from build123d import *

# Parameters (mm, degrees)
MODEL_R                 = 1.5
SALIENTE_EXTRUIR1_DEPTH = 3


with BuildPart() as part:
    # Model → Saliente-Extruir1 (new body)
    with BuildSketch(Plane.XY):
        with BuildLine():
            Line((-105.943383637, 101.056539338), (-105.943383637, 65.056539338))
            ThreePointArc((-105.943383637, 65.056539338), (-104.625364152, 61.874558823), (-101.443383637, 60.556539338))
            Line((-101.443383637, 60.556539338), (-83.443383637, 60.556539338))
            ThreePointArc((-83.443383637, 60.556539338), (-80.261403122, 61.874558823), (-78.943383637, 65.056539338))
            Line((-78.943383637, 65.056539338), (-78.943383637, 101.056539338))
            ThreePointArc((-78.943383637, 101.056539338), (-80.261403122, 104.238519853), (-83.443383637, 105.556539338))
            Line((-83.443383637, 105.556539338), (-101.443383637, 105.556539338))
            ThreePointArc((-101.443383637, 105.556539338), (-104.625364152, 104.238519853), (-105.943383637, 101.056539338))
        make_face()
        with Locations((-101.443383637, 101.056539338)):
            Circle(MODEL_R, mode=Mode.SUBTRACT)
        with Locations((-92.443383637, 101.056539338)):
            Circle(MODEL_R, mode=Mode.SUBTRACT)
        with Locations((-83.443383637, 101.056539338)):
            Circle(MODEL_R, mode=Mode.SUBTRACT)
        with Locations((-101.443383637, 92.056539338)):
            Circle(MODEL_R, mode=Mode.SUBTRACT)
        with Locations((-92.443383637, 92.056539338)):
            Circle(MODEL_R, mode=Mode.SUBTRACT)
        with Locations((-83.443383637, 92.056539338)):
            Circle(MODEL_R, mode=Mode.SUBTRACT)
        with Locations((-101.443383637, 83.056539338)):
            Circle(MODEL_R, mode=Mode.SUBTRACT)
        with Locations((-92.443383637, 83.056539338)):
            Circle(MODEL_R, mode=Mode.SUBTRACT)
        with Locations((-83.443383637, 83.056539338)):
            Circle(MODEL_R, mode=Mode.SUBTRACT)
        with Locations((-101.443383637, 74.056539338)):
            Circle(MODEL_R, mode=Mode.SUBTRACT)
        with Locations((-92.443383637, 74.056539338)):
            Circle(MODEL_R, mode=Mode.SUBTRACT)
        with Locations((-83.443383637, 74.056539338)):
            Circle(MODEL_R, mode=Mode.SUBTRACT)
        with Locations((-101.443383637, 65.056539338)):
            Circle(MODEL_R, mode=Mode.SUBTRACT)
        with Locations((-92.443383637, 65.056539338)):
            Circle(MODEL_R, mode=Mode.SUBTRACT)
        with Locations((-83.443383637, 65.056539338)):
            Circle(MODEL_R, mode=Mode.SUBTRACT)
    extrude(amount=SALIENTE_EXTRUIR1_DEPTH)


solid = part.part
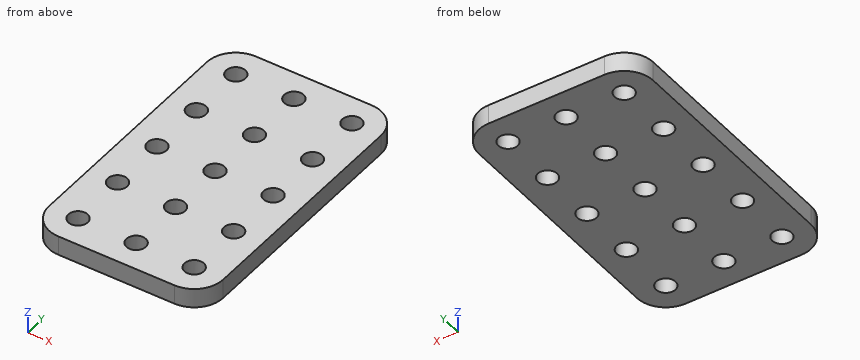
Could you check a few things on this model? Use its own coordinates, in mm. Round coordinates to 2 decimals unless told otherwise and drop trailing zeros. Write each loop counter-clockwise with the first axis right and the second up, starting at its lowest first coordinate (ties: lowest second). Pieces come first, ordered by that corner, then holes. Notation, with made-up numbers: (-18.75, 30.5) -> (-6.75, 30.5) arc R7 cw to (-6.75, 34.5) -> close; hole circle Ø6 at (27.25, -21). An arc over 180 degrees is marked (long way). Use a Markdown table: item, result.
1. If we section it at C-C (z = 1.2): State how many separate pieces and enclosed holes the cut face has, then the cut area to 3 significant figures.
Answer key:
| item | result |
|---|---|
| separate pieces | 1 |
| enclosed holes | 15 |
| area | 1,090 mm^2 |
2. Please list where these lines run through material, in increasing order: probe 1 along X at (y, z) = (65, 2.3); probe 2 along Y at (x, z) = (-91.25, 1.05); probe 3 along X at (y, z) = (100, 1.8).
Answer key:
| item | result |
|---|---|
| probe 1 | x = -105.94 to -102.94, -99.94 to -93.94, -90.94 to -84.94, -81.94 to -78.94 |
| probe 2 | y = 60.56 to 64.15, 65.97 to 73.15, 74.97 to 82.15, 83.97 to 91.15, 92.97 to 100.15, 101.97 to 105.56 |
| probe 3 | x = -105.94 to -102.51, -100.38 to -93.51, -91.38 to -84.51, -82.38 to -78.94 |
3. If we section it at A-A (y = 102): List the corners of the cut face in (x, z) for me, then the cut area to 3 significant figures.
Answer key:
| item | result |
|---|---|
| outline | (-105.84, 0) -> (-102.61, 0) -> (-102.61, 3) -> (-105.84, 3) -> close; (-100.28, 0) -> (-93.61, 0) -> (-93.61, 3) -> (-100.28, 3) -> close; (-91.28, 0) -> (-84.61, 0) -> (-84.61, 3) -> (-91.28, 3) -> close; (-82.28, 0) -> (-79.04, 0) -> (-79.04, 3) -> (-82.28, 3) -> close |
| area | 59.4 mm^2 |
4. If we section it at D-D (y = 91.5): List the corners of the cut face in (x, z) for me.
Answer key:
| item | result |
|---|---|
| outline | (-105.94, 0) -> (-102.84, 0) -> (-102.84, 3) -> (-105.94, 3) -> close; (-100.05, 0) -> (-93.84, 0) -> (-93.84, 3) -> (-100.05, 3) -> close; (-91.05, 0) -> (-84.84, 0) -> (-84.84, 3) -> (-91.05, 3) -> close; (-82.05, 0) -> (-78.94, 0) -> (-78.94, 3) -> (-82.05, 3) -> close |
5. For pin 1 Ø3.5 at (x, y) = (-92.44, 74.06) entering from -Z, with a flat end and sliding along its axis, tell me the tip position at first contact or that it passes through.
Answer key:
| item | result |
|---|---|
| pin 1 | stops at z = 0 |
6. If we section it at B-B (x = -82.75): List the corners of the cut face in (y, z) for me, then the cut area to 3 significant figures.
Answer key:
| item | result |
|---|---|
| outline | (60.61, 0) -> (63.73, 0) -> (63.73, 3) -> (60.61, 3) -> close; (66.39, 0) -> (72.73, 0) -> (72.73, 3) -> (66.39, 3) -> close; (75.39, 0) -> (81.73, 0) -> (81.73, 3) -> (75.39, 3) -> close; (84.39, 0) -> (90.73, 0) -> (90.73, 3) -> (84.39, 3) -> close; (93.39, 0) -> (99.73, 0) -> (99.73, 3) -> (93.39, 3) -> close; (102.39, 0) -> (105.5, 0) -> (105.5, 3) -> (102.39, 3) -> close |
| area | 94.8 mm^2 |
